Design review of the part built by this model. Coordinates are the model's own, in mm. Coordinates: 2 decimals unless noted, no trailing zeros. Write each loop counter-clockwise with the first axis right and the second up, starting at its lowest first coordinate (ties: lowest second). Pieces come first, ordered by that corner, then holes. Notation, with made-up numbers: (-40, -30) - (3, -30) arc R12 ccw to (3, -26) - close; hole circle Ø10 at (39, 69). An arc over 180 degrees is marked (long way). Answer as a JSON object with one key per item and string values.
Autodesk Inventor part; units mm, degrees
ref_plane "YZ Plane" through (0, 0, 0) normal (1, 0, 0) x (0, 1, 0)
ref_plane "XZ Plane" through (0, 0, 0) normal (0, 1, 0) x (-1, 0, 0)
ref_plane "XY Plane" through (0, 0, 0) normal (0, 0, 1) x (1, 0, 0)
sketch "Sketch1" plane through (0, 0, 0) normal (0, 0, 1) x (1, 0, 0)
  line L0 (0, 0) -> (-38.1, 0)
  line L1 (0, 0) -> (0, 95.25)
  line L2 (-6.35, 101.6) -> (-38.1, 101.6)
  line L3 (-38.1, 95.25) -> (-38.1, 0)
  line L4 (-31.75, 101.6) -> (-31.75, 101.6)
  line L5 (-31.75, 101.6) -> (-31.75, 12.7)
  line L6 (0, 101.6) -> (-6.35, 101.6)
  line L7 (-6.35, 101.6) -> (-6.35, 12.7)
  circle A0 centre (-31.75, 12.7) radius 2.1463
  circle A1 centre (-6.35, 12.7) radius 2.1463
  arc A2 (-31.75, 101.6) -> (-38.1, 95.25) centre (-31.75, 95.25) ccw
  arc A3 (0, 95.25) -> (-6.35, 101.6) centre (-6.35, 95.25) ccw
  line L8 (-22.225, 101.6) -> (-22.225, 76.2)
  dimension "d0" = 38.1
  dimension "d1" = 101.6
  dimension "d2" = 6.35
  dimension "d3" = 88.9
  dimension "d4" = 6.35
  dimension "d5" = 4.2926
  dimension "d6" = 4.2926
  dimension "d7" = 88.9
  dimension "d19" = 6.35
  dimension "d20" = 6.35
  dimension "d23" = 25.4
extrude "Plate1" add sketch "Sketch1" along normal blind 6.35
sketch "Sketch4" plane through (0, 0, 0) normal (0, 0, -1) x (-1, 0, 0)
  line L0 (6.35, 101.6) -> (31.75, 101.6)
  line L1 (19.05, 101.6) -> (19.05, 82.55)
  circle A0 centre (19.05, 82.55) radius 14.2875
  dimension "d25" = 19.05
  dimension "d26" = 28.575
extrude "Cut1" cut sketch "Sketch4" against normal blind 6.35
equation "\"d27\" = Thickness"
equation "\"BendRadius\" = Thickness"
equation "\"BendReliefWidth\" = Thickness"
equation "\"BendReliefDepth\" = 0.5 * Thickness"
equation "\"CornerReliefSize\" = 4 * Thickness"
equation "\"MinimumRemnant\" = 2 * Thickness"
equation "\"TransitionRadius\" = BendRadius"
equation "\"JacobiRadiusSize\" = BendRadius"
equation "\"GapSize\" = Thickness"
equation "\"d8\" = BendRadius"
properties part number "arm mount"
(1) Take a section at C-C, the plane z = 1. Give the number of separate pieces and of enclosed holes in the cut face, and give its area (3 significant figures).
Solved:
{"separate pieces": "1", "enclosed holes": "3", "area": "3,180 mm^2"}
(2) To check wall thickness, follow line 1 (X direction, y = 12.7, z = 4.5); line 2 (Y direction, x = -19.05, z = 1.5); line 3 (X direction, y = 82.55, z = 3.25). State the ranges of each line that lie inside material, in increasing order. Write a range as from..to.
Solved:
{"line 1": "x = -38.1..-33.9, -29.6..-8.5, -4.2..0", "line 2": "y = 0..68.26, 96.84..101.6", "line 3": "x = -38.1..-33.34, -4.76..0"}
(3) Take a section at A-A, the plane x = -19.05. Write out the cut boundary in (y, z), and give its area (3 significant figures).
Solved:
{"outline": "(0, 0) - (68.26, 0) - (68.26, 6.35) - (0, 6.35) - close; (96.84, 0) - (101.6, 0) - (101.6, 6.35) - (96.84, 6.35) - close", "area": "464 mm^2"}
(4) The part is to be moulded in two halves that separate along X. For faces 1 (the face through (-19, 0, 3)), 2 (the face through (-36.29, 99.69, 3.13)), 3 (the face through (-6.8, 14.8, 3.1)), say which applies: pulls with the +X half, pulls with the -X half, needs draft (parallel to the pull), parting line crosses it, or undercut.
Solved:
{"face 1": "needs draft", "face 2": "pulls with the -X half", "face 3": "undercut"}
(5) For pin 1 (2.5 mm diameter, centred on x = -6.35, y = 12.7, fed in from -Z), flat-tipped, find the tip position at first contact; note if it passes through.
Solved:
{"pin 1": "passes through"}
(6) Take a section at B-B, the plane y = 82.55. Write out the cut boundary in (x, z).
Solved:
{"outline": "(-38.1, 0) - (-33.34, 0) - (-33.34, 6.35) - (-38.1, 6.35) - close; (-4.76, 0) - (0, 0) - (0, 6.35) - (-4.76, 6.35) - close"}
